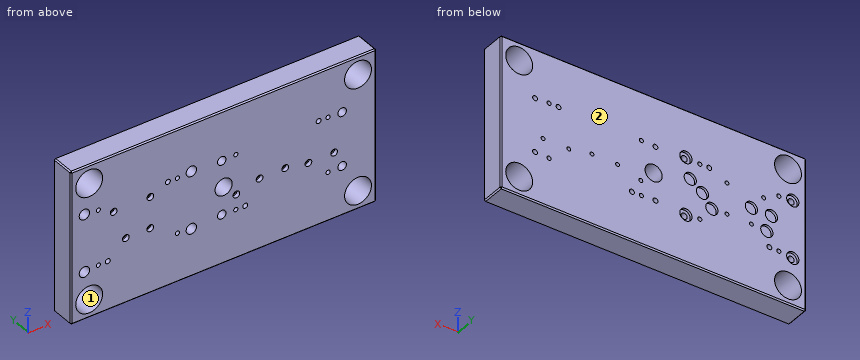
```python
from build123d import *

# Parameters (mm, degrees)
SKETCH2_W                                           = 500
SKETCH2_H                                           = 125
BOSS_EXTRUDE1_DEPTH                                 = 40
SKETCH3_W                                           = 500
SKETCH3_H                                           = 40
BOSS_EXTRUDE2_DEPTH                                 = 125
SKETCH6_R                                           = 22
CUT_EXTRUDE1_DEPTH                                  = 316.04959927
M30X2_0_TAPPED_HOLE1_D                              = 28
CHAMFER1_SIZE                                       = 2
M8_TAPPED_HOLE1_D                                   = 6.8
F_8_0MM_DOWEL_HOLE1_D                               = 8
CBORE_FOR_M6_HEX_SOCKET_HEAD_CAP_SCREW1_D           = 6.4
CBORE_FOR_M6_HEX_SOCKET_HEAD_CAP_SCREW1_CBORE_D     = 11
CBORE_FOR_M6_HEX_SOCKET_HEAD_CAP_SCREW1_CBORE_DEPTH = 6.4
CBORE_FOR_M6_HEX_SOCKET_HEAD_CAP_SCREW2_D           = 6.4
CBORE_FOR_M6_HEX_SOCKET_HEAD_CAP_SCREW2_CBORE_D     = 11
CBORE_FOR_M6_HEX_SOCKET_HEAD_CAP_SCREW2_CBORE_DEPTH = 6.4
SKETCH25_R                                          = 10
CUT_EXTRUDE2_DEPTH                                  = 4
F_10_0_10_DIAMETER_HOLE1_D                          = 10
SKETCH35_R                                          = 8.5
CUT_EXTRUDE3_DEPTH                                  = 24
F_8_0_8_DIAMETER_HOLE2_D                            = 8
SKETCH43_R                                          = 7
CUT_EXTRUDE4_DEPTH                                  = 32


with BuildPart() as part:
    # Sketch2 → Boss-Extrude1 (new body)
    with BuildSketch(Plane(origin=(0, 0, 0), x_dir=(1, 0, 0), z_dir=(0, 1, 0))):
        Rectangle(SKETCH2_W, SKETCH2_H)
    extrude(amount=BOSS_EXTRUDE1_DEPTH)

    # Sketch3 → Boss-Extrude2 (add)
    with BuildSketch(Plane(origin=(0, 0, -62.5), x_dir=(-1, 0, 0), z_dir=(0, 0, -1))):
        with Locations((0, 20)):
            Rectangle(SKETCH3_W, SKETCH3_H)
    extrude(amount=BOSS_EXTRUDE2_DEPTH)

    # Sketch6 → Cut-Extrude1 (cut, through all)
    with BuildSketch(Plane(origin=(0, 0, 0), x_dir=(-1, 0, 0), z_dir=(0, -1, 0))):
        with Locations(Location((-220, 157.5, 0), (0, 0, 90))):
            Circle(SKETCH6_R)
        with Locations(Location((-220, -32.5, 0), (0, 0, 90))):
            Circle(SKETCH6_R)
    cut_extrude1 = extrude(amount=-CUT_EXTRUDE1_DEPTH, mode=Mode.SUBTRACT)

    # Mirror1: Cut-Extrude1 across plane
    add(cut_extrude1.mirror(Plane(origin=(0, 0, 0), x_dir=(0, 0, 1), z_dir=(1, 0, 0))), mode=Mode.SUBTRACT)

    # M30x2.0 Tapped Hole1 (through all)
    with Locations(Plane(origin=(0, 40, 0), x_dir=(1, 0, 0), z_dir=(0, 1, 0))):
        with Locations((0, 62.5)):
            Hole(M30X2_0_TAPPED_HOLE1_D / 2)

    # Chamfer1
    chamfer1_edges = [part.edges().sort_by_distance(p)[0] for p in [
        (-250, 40, -62.5),
        (0, 40, -187.5),
        (0, 40, 62.5),
        (250, 20, -187.5),
        (0, 0, -187.5),
        (-250, 20, -187.5),
        (250, 40, -62.5),
        (0, 0, 62.5),
        (-250, 0, -62.5),
        (250, 0, -62.5),
        (250, 20, 62.5),
        (-250, 20, 62.5),
    ]]
    chamfer(chamfer1_edges, length=CHAMFER1_SIZE)

    # M8 Tapped Hole1 (through all)
    with Locations(Plane(origin=(0, 0, 0), x_dir=(-1, 0, 0), z_dir=(0, -1, 0))):
        with Locations((-171, 17.5), (-19.969, 17.5), (-19.969, 107.5), (-171, 107.5), (75.632503002, 107.5), (205, 107.5), (205, 17.5), (75.632503002, 17.5)):
            Hole(M8_TAPPED_HOLE1_D / 2)

    # Ø8.0mm Dowel Hole1 (through all)
    with Locations(Plane(origin=(0, 0, 0), x_dir=(-1, 0, 0), z_dir=(0, -1, 0))):
        with Locations((-155.5, 17.5), (-35.469, 107.5), (91.132503002, 17.258975019), (189.5, 107.228378806)):
            Hole(F_8_0MM_DOWEL_HOLE1_D / 2)

    # CBORE for M6 Hex Socket Head Cap Screw1 (through all)
    with Locations(Plane(origin=(0, 0, 0), x_dir=(-1, 0, 0), z_dir=(0, -1, 0))):
        with Locations((-180.875, 79.28), (-100.875, 72.352366083), (-58.875, 72.352366083), (-20.875, 83.19101), (-138.875, 79.28)):
            CounterBoreHole(CBORE_FOR_M6_HEX_SOCKET_HEAD_CAP_SCREW1_D / 2, CBORE_FOR_M6_HEX_SOCKET_HEAD_CAP_SCREW1_CBORE_D / 2, CBORE_FOR_M6_HEX_SOCKET_HEAD_CAP_SCREW1_CBORE_DEPTH)

    # CBORE for M6 Hex Socket Head Cap Screw2 (through all)
    with Locations(Plane(origin=(0, 0, 0), x_dir=(-1, 0, 0), z_dir=(0, -1, 0))):
        with Locations((160, 81.36), (120.125, 81.36), (120, 30.34), (180, 30.34)):
            CounterBoreHole(CBORE_FOR_M6_HEX_SOCKET_HEAD_CAP_SCREW2_D / 2, CBORE_FOR_M6_HEX_SOCKET_HEAD_CAP_SCREW2_CBORE_D / 2, CBORE_FOR_M6_HEX_SOCKET_HEAD_CAP_SCREW2_CBORE_DEPTH)

    # Sketch25 → Cut-Extrude2 (cut)
    with BuildSketch(Plane(origin=(0, 40, 0), x_dir=(1, 0, 0), z_dir=(0, 1, 0))):
        with Locations(Location((-227.816251501, 15.5, 0), (0, 0, 270))):
            Circle(SKETCH25_R)
        with Locations(Location((-52.816251501, 15.5, 0), (0, 0, 270))):
            Circle(SKETCH25_R)
        with Locations(Location((-52.816251501, 109.5, 0), (0, 0, 270))):
            Circle(SKETCH25_R)
        with Locations(Location((-227.816251501, 109.5, 0), (0, 0, 270))):
            Circle(SKETCH25_R)
        with Locations(Location((-185.316251501, 82.5, 0), (0, 0, 270))):
            Circle(SKETCH25_R)
        with Locations(Location((-192.816251501, 54.78, 0), (0, 0, 270))):
            Circle(SKETCH25_R)
        with Locations(Location((-160, 54.78, 0), (0, 0, 270))):
            Circle(SKETCH25_R)
        with Locations(Location((-95.316251501, 82.5, 0), (0, 0, 270))):
            Circle(SKETCH25_R)
        with Locations(Location((-80, 62.78, 0), (0, 0, 270))):
            Circle(SKETCH25_R)
        with Locations(Location((-60, 47.78, 0), (0, 0, 270))):
            Circle(SKETCH25_R)
    extrude(amount=-CUT_EXTRUDE2_DEPTH, mode=Mode.SUBTRACT)

    # Ø10.0 (10) Diameter Hole1 (through all)
    with Locations(Plane(origin=(0, 40, 0), x_dir=(1, 0, 0), z_dir=(0, 1, 0))):
        with Locations((-52.816251501, 15.5), (-227.816251501, 109.5), (-227.816251501, 15.5), (-52.816251501, 109.5)):
            Hole(F_10_0_10_DIAMETER_HOLE1_D / 2)

    # Sketch35 → Cut-Extrude3 (cut)
    with BuildSketch(Plane.XZ):
        with Locations(Location((-52.816251501, -109.5, 0), (0, 0, 270))):
            Circle(SKETCH35_R)
        with Locations(Location((-227.816251501, -15.5, 0), (0, 0, 270))):
            Circle(SKETCH35_R)
        with Locations(Location((-227.816251501, -109.5, 0), (0, 0, 270))):
            Circle(SKETCH35_R)
        with Locations(Location((-52.816251501, -15.5, 0), (0, 0, 270))):
            Circle(SKETCH35_R)
    extrude(amount=-CUT_EXTRUDE3_DEPTH, mode=Mode.SUBTRACT)

    # Ø8.0 (8) Diameter Hole2 (through all)
    with Locations(Plane(origin=(0, 40, 0), x_dir=(1, 0, 0), z_dir=(0, 1, 0))):
        with Locations((-3.031, 106.5), (-3.031, 18.5), (194, 106.5), (194, 18.5)):
            Hole(F_8_0_8_DIAMETER_HOLE2_D / 2)

    # Sketch43 → Cut-Extrude4 (cut)
    with BuildSketch(Plane.XZ):
        with Locations(Location((194, -106.5, 0), (0, 0, 270))):
            Circle(SKETCH43_R)
        with Locations(Location((194, -18.5, 0), (0, 0, 270))):
            Circle(SKETCH43_R)
        with Locations(Location((-3.031, -18.5, 0), (0, 0, 270))):
            Circle(SKETCH43_R)
        with Locations(Location((-3.031, -106.5, 0), (0, 0, 270))):
            Circle(SKETCH43_R)
    extrude(amount=-CUT_EXTRUDE4_DEPTH, mode=Mode.SUBTRACT)


solid = part.part
```
Model file for the job. Use its own axes, mm. Face numbers are marked on the shaded views. Round coordinates to 2 decimals unless told otherwise and drop trailing zeros. Write each loop counter-clockwise with the first axis right and the second up, starting at its lowest first coordinate (ties: lowest second). Pieces come first, ordered by that corner, then holes. Notation, with made-up numbers: (51, 41) -> (88, 41) arc R11 cw to (88, 52) -> close; hole circle Ø1 at (5.25, -26). An arc over 180 degrees is marked (long way). Answer as CSV lines item,"result".
1. Drill centre lines: line 1 (Z direction, x = -120, y = 20); line 2 (X direction, y = 27.5, z = -30.34); line 3 (Z direction, x = -180, y = 23). Where is each one in solid material? Low to high.
Resolved:
line 1,"-187.5 to -84.56, -78.16 to -33.54, -27.14 to 62.5"
line 2,"-250 to -183.2, -176.8 to -123.2, -116.8 to 250"
line 3,"-187.5 to -33.54, -27.14 to 62.5"
2. Mould opens along X. For the marked faces 1 and 2 say: +X half, -X half, draft (parallel to the pull), parting line (faces both ways), or undercut.
Resolved:
face 1,"undercut"
face 2,"draft"
3. Slice it at B-B, the plane x = 211. List the corners of the cut face in (y, z), plus the area to 3 significant figures.
Resolved:
outline,"(0, -185.5) -> (2, -187.5) -> (38, -187.5) -> (40, -185.5) -> (40, -177.57) -> (0, -177.57) -> close; (0, -137.43) -> (40, -137.43) -> (40, 12.43) -> (0, 12.43) -> close; (0, 52.57) -> (40, 52.57) -> (40, 60.5) -> (38, 62.5) -> (2, 62.5) -> (0, 60.5) -> close"
area,"6,780 mm²"
4. Slice it at A-A, the plane z = -157.5. List the corners of the cut face in (x, y).
Resolved:
outline,"(-250, 2) -> (-248, 0) -> (-242, 0) -> (-242, 40) -> (-248, 40) -> (-250, 38) -> close; (-198, 0) -> (198, 0) -> (198, 40) -> (-198, 40) -> close; (242, 0) -> (248, 0) -> (250, 2) -> (250, 38) -> (248, 40) -> (242, 40) -> close"
5. Pin check, flat tips, straight feed: pin 1 Ø12 at (x, z) = (-52.82, -15.5) entering from +Y; pin 2 Ø6.5 at (x, z) = (194, -18.5) entering from +Y; pin 3 Ø16 at (x, z) = (-227.82, -15.5) entering from -Y. Stop position of each tip, or through.
Resolved:
pin 1,"y = 36"
pin 2,"through"
pin 3,"y = 24"
